```python
from build123d import *

# Parameters (mm, degrees)
SKETCH_1_R      = 3.999999996
SKETCH_1_R_2    = 4
EXTRUDE_1_DEPTH = 5.5


with BuildPart() as part:
    # Эскиз1 → Вытянуть1 (new body)
    with BuildSketch(Plane(origin=(0, 0, 0), x_dir=(0, 0, -1), z_dir=(1, 0, 0))):
        with BuildLine():
            ThreePointArc((-9.540871081, -26.398646507), (-2.597990728, -7.694762203), (-20.375077368, 1.361399581))
            add(Edge.make_bspline(
                [(-20.375077368, 1.361399581), (-59.744347093, -6.195572957), (-142.43517779, -71.38922898), (-60.423943676, -114.845698035)],
                knots=[0, 0, 0, 0, 1, 1, 1, 1], degree=3))
            ThreePointArc((-60.423943676, -114.845698035), (-39.682689443, -108.483068728), (-47.637725769, -88.298914648))
            add(Edge.make_bspline(
                [(-9.540871081, -26.398646507), (-57.761471468, -47.925661264), (-93.927707693, -72.902178799), (-47.637725769, -88.298914648)],
                knots=[0, 0, 0, 0, 1, 1, 1, 1], degree=3))
        make_face()
        with Locations((-16.571481544, -13.148344)):
            Circle(SKETCH_1_R, mode=Mode.SUBTRACT)
        with Locations((-52.996333561, -102.070572255)):
            Circle(SKETCH_1_R_2, mode=Mode.SUBTRACT)
    extrude(amount=EXTRUDE_1_DEPTH)


solid = part.part
```
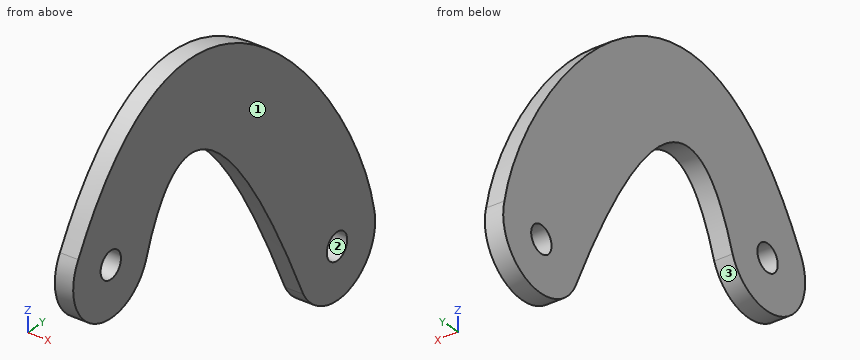
Verification items for the finished model (mm, model axes). Face numbers are marked on the shaded views. Round coordinates to 2 decimals unless told otherwise and drop trailing zeros. Answer as a JSON object with one key per item and string values. Group by question number.
Q1. Mould release check, pull along Z, two halves, no side actions. Record for the marked faces 1, 2 and 3: released by +Z, released by -Z, zero draft, split by the parting line, or undercut.
Q2. Go/stop test with flat-tipped pins: pin 1 Ø1.5 at (x, z) = (3, 52) entering from -Y; pin 2 Ø2 at (x, z) = (4, 52.5) entering from +Y; pin 3 Ø9 at (y, z) = (-102.07, 53) entering from -X; pin 4 Ø5 at (y, z) = (-13.15, 16.57) entering from -X. Record where each tip stops, or that it passes through.
Q3. Thickness scan on line 1 (Y direction, x = 5.15, z = 51.5); line 2 (Y direction, x = 1.5, z = 53.5); line 3 (Z direction, x = 4.3, y = -103). Record the ranges inside material, lowest first.
Q4. Section check A-A, the plane x = 1.85. Give the number of separate pieces and of enclosed holes in the cut face, plus the area to 3 significant figures.
Found:
{
 "1": {"face 1": "zero draft", "face 2": "undercut", "face 3": "split by the parting line"},
 "2": {"pin 1": "stops at y = -116.85", "pin 2": "stops at y = -11.8", "pin 3": "stops at x = 0", "pin 4": "passes through"},
 "3": {"line 1": "y = -116.77 to -105.78, -98.36 to -86.92, -48.85 to -11.8", "line 2": "y = -116.84 to -106.04, -98.1 to -86.12, -50.27 to -13.05", "line 3": "z = 38.25 to 49.11, 56.89 to 78.3"},
 "4": {"separate pieces": "1", "enclosed holes": "2", "area": "4,540 mm^2"}
}
